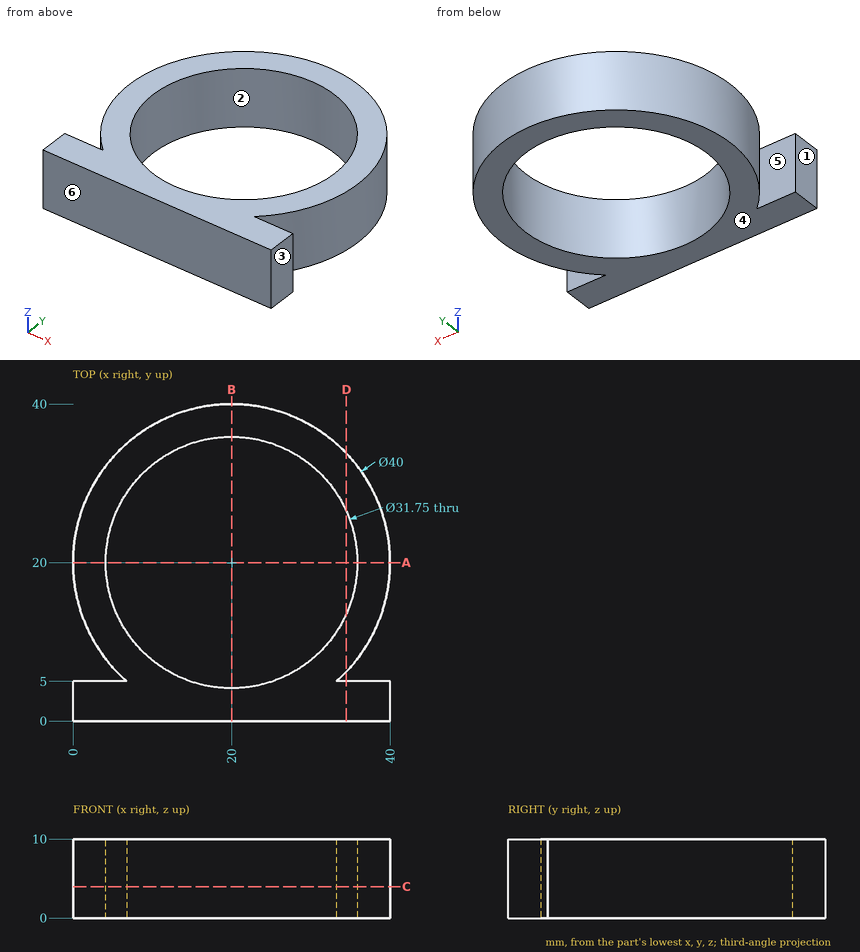
Design review of the part shown in the three views and the two pictorial views. Dimensions are in mm from the part's minimum x, y and z. A direction names the side the tool comes from. Give positions to 0.01 mm unless a question says otherwise; leave off trailing zeros. Write each loop counter-clockwise with the first axis right and the second up, starting at its lowest first coordinate (ties: lowest second). Pieces come first, ordered by that corner, then holes. Notation, with made-up numbers: M 43,60.25 L 47,60.25 A7 ccw 47,66.25 Z; hole C -2,52.25 d3. An arc over 180 degrees is marked long. Return JSON: item names as keys, results as strings. Group by question number.
Item 1: Take a section at A-A (y = 20). Give the boundary of the cut face in (x, z) (3 decimals), plus the area to 3 significant figures.
Item 2: Wall thickness on line 1 along Y through (x, z) = (20, 6.75) (3 decimals); line 2 along X through (y, z) = (19.5, 7.25); line 3 along Y through (x, z) = (16, 3.75): over which ranges is each line inside the solid? List them lowest first.
Item 3: Clearance check with flat-ended pins moving along their axes: pin 1 Ø4 at (x, z) = (5.5, 5.5) entering from +Y; pin 2 Ø6 at (x, y) = (30, 22) entering from +Z; pin 3 Ø2 at (x, z) = (36, 5) entering from +Y; pin 4 Ø1 at (x, z) = (17, 6.5) entering from +Y. State where each tip first meets the part, or that it passes through.
Item 4: Tool access review of the marked faces 5 and 6: name each direction out of +Z, -Z, +X, -X, +Y, -Y from which nothing blocks a thin tool from reaching the whole face with its end or side.
Item 5: Take a section at D-D (x = 34.5). Give the boundary of the cut face in (y, z), plus the area to 3 significant figures.
Item 6: The part is to be moulded in two halves that separate along X. For the marked faces 1, 2, 3 and 4, say which applies: pulls with the +X half, pulls with the -X half, needs draft (parallel to the pull), parting line crosses it, or undercut.
Item 7: Take a section at C-C (z = 4). Give the boundary of the cut face in (x, y) (3 decimals), plus the area to 3 significant figures.
Return value:
{
 "1": {"outline": "M 0,0 L 4.125,0 L 4.125,10 L 0,10 Z; M 35.875,0 L 40,0 L 40,10 L 35.875,10 Z", "area": "82.5 mm2"},
 "2": {"line 1": "y = 0 to 4.125, 35.875 to 40", "line 2": "x = 0.01 to 4.13, 35.87 to 39.99", "line 3": "y = 0 to 4.64, 35.36 to 39.6"},
 "3": {"pin 1": "stops at y = 35.61", "pin 2": "passes through", "pin 3": "stops at y = 33.23", "pin 4": "stops at y = 39.84"},
 "4": {"face 5": "+Z, -Z, -X", "face 6": "+Z, -Z, +X, -X, -Y"},
 "5": {"outline": "M 0,0 L 5,0 L 5,10 L 0,10 Z; M 6.23,0 L 13.54,0 L 13.54,10 L 6.23,10 Z; M 26.46,0 L 33.77,0 L 33.77,10 L 26.46,10 Z", "area": "196 mm2"},
 "6": {"face 1": "pulls with the -X half", "face 2": "undercut", "face 3": "pulls with the +X half", "face 4": "needs draft"},
 "7": {"outline": "M 0,0 L 40,0 L 40,5 L 33.229,5 A20 ccw long 6.771,5 L 0,5 Z; hole C 20,20 d31.75", "area": "574 mm2"}
}
